```python
from build123d import *
from build123d.topology import SkipClean

# Parameters (mm, degrees)
BOSS_EXTRUDE2_DEPTH = 20
FILLET1_R           = 10
CHAMFER1_SIZE       = 1
SKETCH2_R           = 1.5
CUT_EXTRUDE1_DEPTH  = 20
CHAMFER3_SIZE       = 1


with BuildPart() as part:
    # Sketch1 → Boss-Extrude2 (new body)
    with BuildSketch(Plane.XY):
        with BuildLine():
            Line((138.685446009, 16.430118313), (158.685446009, 16.430118313))
            Line((158.685446009, 16.430118313), (188.685446009, 16.430118313))
            Line((188.685446009, 16.430118313), (188.685446009, 26.430118313))
            Line((188.685446009, 26.430118313), (158.685446009, 26.430118313))
            Line((158.685446009, 26.430118313), (158.685446009, 216.430118313))
            Line((158.685446009, 216.430118313), (138.685446009, 216.430118313))
            Line((138.685446009, 216.430118313), (138.685446009, 201.505118313))
            ThreePointArc((138.685446009, 201.505118313), (143.760446009, 196.430118313), (138.685446009, 191.355118313))
            Line((138.685446009, 191.355118313), (138.685446009, 16.430118313))
        make_face()
    extrude(amount=BOSS_EXTRUDE2_DEPTH)

    # Fillet1
    fillet1_edges = [part.edges().sort_by_distance(p)[0] for p in [
        (158.685446009, 26.430118313, 10),
    ]]
    fillet(fillet1_edges, radius=FILLET1_R)

    # Chamfer1
    chamfer1_edges = [part.edges().sort_by_distance(p)[0] for p in [
        (158.685446009, 216.430118313, 10),
        (188.685446009, 26.430118313, 10),
    ]]
    chamfer(chamfer1_edges, length=CHAMFER1_SIZE)

    # Sketch2 → Cut-Extrude1 (cut)
    with BuildSketch(Plane(origin=(0, 26.430118313, 0), x_dir=(1, 0, 0), z_dir=(0, 1, 0))):
        with Locations(Location((178.185446009, -5.5, 0), (0, 0, 270))):
            Circle(SKETCH2_R)
        with Locations(Location((178.185446009, -14.5, 0), (0, 0, 270))):
            Circle(SKETCH2_R)
    extrude(amount=-CUT_EXTRUDE1_DEPTH, mode=Mode.SUBTRACT)

    # Chamfer3
    chamfer3_edges = [part.edges().sort_by_distance(p)[0] for p in [
        (178.185446009, 26.430118313, 4),
        (178.185446009, 26.430118313, 13),
    ]]
    chamfer(chamfer3_edges, length=CHAMFER3_SIZE)

    # Mirror1: part across plane


with BuildPart() as part_1:
    with SkipClean():  # the faces are left unmerged after this step: merging them gives an invalid solid
        add(part.part)
        add(part.part.mirror(Plane(origin=(138.685446009, 16.430118313, 20), x_dir=(0, 0, 1), z_dir=(1, 0, 0))))


solid = part_1.part
```
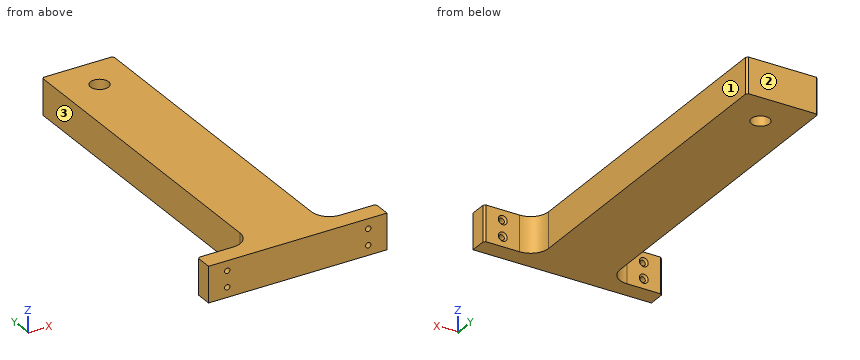
Source: CAD feature listing. Evaluate the final solid. Frame: model axes, mm. Face numbers are marked on the shaded views. A direction names the side the tool comes from. Round coordinates to 2 decimals unless told otherwise and drop trailing zeros. Loops run counter-clockwise (first coordinate to the right, second up) from the corner with the lowest first, then second, coordinate; pieces in that order, holes last. Notation, with made-up numbers: M 22,-38 L 48,-38 A23 ccw 48,1 Z; hole C 16,18 d5. An arc over 180 degrees is marked long. Use a Markdown table: item, result. Add a question column.
1. Section query A-A on z = 10. Return the cut outline in (x, y) (3 decimals).
2. Section query B-B on y = 86.5. Return the cut outline in (x, z).
3. Reachability of the marked faces 1, 2 and 3 from +Z, -Z, +X, -X, +Y, -Y: full face, straight path, thin tool, end or side. Return the list, or none.
4. Section query C-C on x = 106.5. Return the cut outline in (y, z).
5. Line query: line 1 (X direction, y = 23.75, z = 5.5); line 2 (X direction, y = 57, z = 14); line 3 (Y direction, x = 172, z = 15). Output: solid intervals per line, ascending.
6. Contact query for flat-ended pins moving along their axis: P1, Ø1.8, axis at x = 178.19, z = 14.5, coming from the +Y side; P2, Ø9.5, axis at x = 178, z = 14, coming from the +Y side; P3, Ø6, axis at y = 112.5, z = 13.5, coming from the -X side; P4, Ø4, axis at y = 116, z = 10, coming from the +X side. Output: stop coordinate, or through.
Reported:
| question | item | result |
|---|---|---|
| 1 | outline | M 88.685,16.43 L 188.685,16.43 L 188.685,25.43 L 187.685,26.43 L 168.685,26.43 A10 cw 158.685,36.43 L 158.685,215.43 L 157.685,216.43 L 119.685,216.43 L 118.685,215.43 L 118.685,36.43 A10 cw 108.685,26.43 L 89.685,26.43 L 88.685,25.43 Z; hole C 138.685,196.43 d10.15 |
| 2 | outline | M 118.69,0 L 158.69,0 L 158.69,20 L 118.69,20 Z |
| 3 | face 1 | +Z, -Z, +X, +Y |
| 3 | face 2 | +Z, -Z, +X, -X, +Y |
| 3 | face 3 | +Z, -Z, -X, +Y |
| 4 | outline | M 16.43,0 L 26.43,0 L 26.43,20 L 16.43,20 Z |
| 5 | line 1 | x = 88.69 to 97.69, 100.69 to 176.69, 179.69 to 188.69 |
| 5 | line 2 | x = 118.69 to 158.69 |
| 5 | line 3 | y = 16.43 to 26.43 |
| 6 | P1 | passes through |
| 6 | P2 | stops at y = 26.43 |
| 6 | P3 | stops at x = 118.69 |
| 6 | P4 | stops at x = 158.69 |
